Source: CAD feature listing. Evaluate the final solid. Frame: model axes, mm. Give positions to 0.01 mm unless a question says otherwise; leave off trailing zeros. Loops run counter-clockwise (first coordinate to the right, second up) from the corner with the lowest first, then second, coordinate; pieces in that order, holes last.
from build123d import *

# Parameters (mm, degrees)
BASE_EXTRUDE_THIN_DEPTH = 2197.1
INSIDE_BEND_RADIUS_R    = 12.7
OUTSIDE_BEND_RADIUS_R   = 22.225


with BuildPart() as part:
    # Sketch1 → Base-Extrude-Thin (new body)
    with BuildSketch(Plane.XY):
        Polygon((-88.9, 0), (0, 0), (0, 260.35), (-88.9, 260.35), (-88.9, 250.825), (-9.525, 250.825), (-9.525, 9.525), (-88.9, 9.525), align=None)
    extrude(amount=-BASE_EXTRUDE_THIN_DEPTH)

    # Inside Bend Radius
    inside_bend_radius_edges = [part.edges().sort_by_distance(p)[0] for p in [
        (-9.525, 250.825, -1098.55),
        (-9.525, 9.525, -1098.55),
    ]]
    fillet(inside_bend_radius_edges, radius=INSIDE_BEND_RADIUS_R)

    # Outside Bend Radius
    outside_bend_radius_edges = [part.edges().sort_by_distance(p)[0] for p in [
        (0, 0, -1098.55),
        (0, 260.35, -1098.55),
    ]]
    fillet(outside_bend_radius_edges, radius=OUTSIDE_BEND_RADIUS_R)


solid = part.part
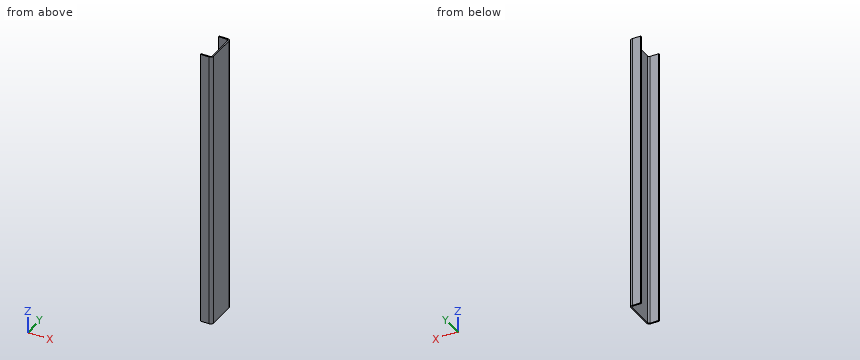
1) Cut plane A-A (x = -69.5). Return loops of the section in (y, z) (3 decimals).
Checks:
outline: (0, -2197.1) - (9.525, -2197.1) - (9.525, 0) - (0, 0) - close; (250.825, -2197.1) - (260.35, -2197.1) - (260.35, 0) - (250.825, 0) - close
2) Cut plane B-B (z = -1862.5). Return loops of the section in (x, y) (3 decimals).
Checks:
outline: (-88.9, 0) - (-22.225, 0) arc R22.225 ccw to (0, 22.225) - (0, 238.125) arc R22.225 ccw to (-22.225, 260.35) - (-88.9, 260.35) - (-88.9, 250.825) - (-22.225, 250.825) arc R12.7 cw to (-9.525, 238.125) - (-9.525, 22.225) arc R12.7 cw to (-22.225, 9.525) - (-88.9, 9.525) - close
3) Cut plane C-C (y = 56.5). Return loops of the section in (x, z) (3 decimals).
Checks:
outline: (-9.525, -2197.1) - (0, -2197.1) - (0, 0) - (-9.525, 0) - close
4) Contact query for a flat-ended pin moving along its axis: P1, Ø5, axis at y = 82.5, z = -1369.5, coming from the -X side (3 decimals). Output: stop coordinate, or through.
Checks:
P1: stops at x = -9.525
5) Ray query, probe 1 along Y at (x, z) = (-23.5, -748) (3 decimals); probe 2 along X at (y, z) = (93, -343) (3 decimals); probe 3 along Y at (x, z) = (-21, -1399). Return the intervals inside material, ascending.
Checks:
probe 1: y = 0 to 9.525, 250.825 to 260.35
probe 2: x = -9.525 to 0
probe 3: y = 0.03 to 9.58, 250.77 to 260.32
